Part model, mm, in its own coordinate system. Face numbers are marked on the shaded views. A direction names the side the tool comes from. Round coordinates to 2 decimals unless told otherwise and drop trailing zeros. Write each loop counter-clockwise with the first axis right and the second up, starting at its lowest first coordinate (ties: lowest second). Pieces come first, ordered by that corner, then holes.
1) Saw through at D-D on y = 13. Write the cut outline in (x, z), and give its area (3 significant figures).
2) Drill centre lines: L1, parallel to X at y = 6.75, z = 16; L2, parallel to Y at x = 5.15, z = 23; L3, parallel to Y at x = -7.9, z = 23. Where is each one in solid material? Low to high.
3) Saw through at A-A on y = 8.5. Write the cut outline in (x, z).
4) Saw through at B-B on x = 0. Write the cut outline in (y, z).
5) Which spindle directions (+Z, -Z, +X, -X, +Y, -Y) get a long thin tool onto all of the face, cutting with end or side? Do the marked faces 4, 5, 6, 7 and 8. Say none if no direction does.
6) Saw through at C-C on z = 8.5. Write the cut outline in (x, y), and give its area (3 significant figures).
7) Flat gauge pins, fed straight in: pin 1 (7 mm diameter, centred on x = 0, z = 8.5, fed in from -Y); pin 2 (1.5 mm diameter, centred on x = 8, y = 13.5, fed in from -Z); pin 3 (2 mm diameter, centred on y = 13, z = 23, fed in from -X); pin 4 (8 mm diameter, centred on x = 6.5, z = 13, fed in from +Y). Where does each tip first touch, or does it go through?
8) Pull direction X, two halves, no side cores. Call the marked faces 1, 2 and 3: +X half, -X half, draft (parallel to the pull), parting line (faces both ways), or undercut.
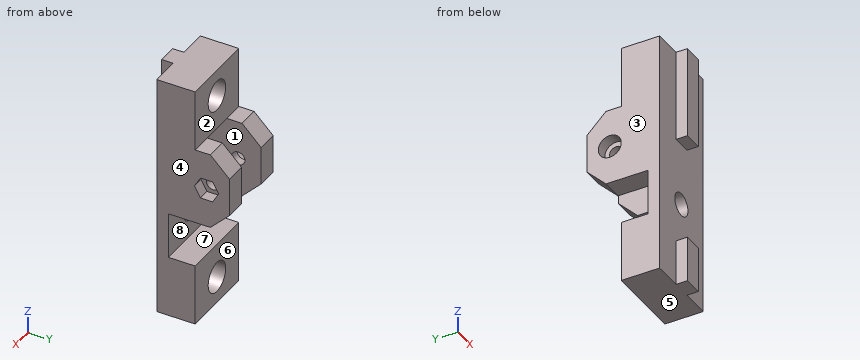
```python
from build123d import *

# Parameters (mm, degrees)
SKETCH1_W               = 20
SKETCH1_H               = 30
BOSS_EXTRUDE1_DEPTH     = 3
SKETCH2_W               = 5
SKETCH2_H               = 12
BOSS_EXTRUDE2_DEPTH     = 3
SKETCH3_R               = 7
SKETCH3_R_2             = 4
BOSS_EXTRUDE3_DEPTH     = 7
SKETCH4_R               = 4
BOSS_EXTRUDE4_DEPTH     = 1
CUT_EXTRUDE1_DEPTH      = 20.339079606
CUT_EXTRUDE1_DEPTH_BACK = 20.339079606
SKETCH5_R               = 3
SKETCH6_R               = 7
SKETCH6_R_2             = 4
BOSS_EXTRUDE6_DEPTH     = 7
SKETCH7_W               = 20
SKETCH7_H               = 3
BOSS_EXTRUDE7_DEPTH     = 19
SKETCH8_W               = 5
SKETCH8_H               = 3
BOSS_EXTRUDE8_DEPTH     = 12
SKETCH10_W              = 5.5
SKETCH10_H              = 20
BOSS_EXTRUDE9_DEPTH     = 16
CUT_EXTRUDE2_DEPTH      = 57.231663678
CUT_EXTRUDE2_DEPTH_BACK = 57.231663678
SKETCH11_R              = 1.75
SKETCH12_R              = 3
SKETCH12_R_2            = 1.75
CUT_EXTRUDE3_DEPTH      = 3
CUT_EXTRUDE4_START      = -3
SKETCH13_R              = 1.75
CUT_EXTRUDE4_DEPTH      = 3
CHAMFER2_SIZE           = 5
CUT_EXTRUDE5_START      = -1.5
SKETCH14_R              = 4
CUT_EXTRUDE5_DEPTH      = 1.5


with BuildPart() as part:
    # Sketch1 → Boss-Extrude1 (new body)
    with BuildSketch(Plane(origin=(0, 0, 0), x_dir=(1, 0, 0), z_dir=(0, 1, 0))):
        Rectangle(SKETCH1_W, SKETCH1_H)
    boss_extrude1 = extrude(amount=BOSS_EXTRUDE1_DEPTH)

    # Sketch2 → Boss-Extrude2 (add)
    with BuildSketch(Plane.XZ):
        with Locations((0, -9)):
            Rectangle(SKETCH2_W, SKETCH2_H)
    boss_extrude2 = extrude(amount=BOSS_EXTRUDE2_DEPTH)

    # Sketch3 → Boss-Extrude3 (add)
    with BuildSketch(Plane(origin=(0, 3, 0), x_dir=(1, 0, 0), z_dir=(0, 1, 0))):
        with Locations(Location((0, 8, 0), (0, 0, 90))):
            Circle(SKETCH3_R)
        with Locations(Location((0, 8, 0), (0, 0, 270))):
            Circle(SKETCH3_R_2, mode=Mode.SUBTRACT)
    boss_extrude3 = extrude(amount=BOSS_EXTRUDE3_DEPTH)

    # Sketch4 → Boss-Extrude4 (add)
    with BuildSketch(Plane(origin=(0, 3, 0), x_dir=(1, 0, 0), z_dir=(0, 1, 0))):
        with Locations(Location((0, 8, 0), (0, 0, 270))):
            Circle(SKETCH4_R)
    boss_extrude4 = extrude(amount=BOSS_EXTRUDE4_DEPTH)

    # Sketch5 → Cut-Extrude1 (cut, two sides: drawn at the far end of the back side and taken through both)
    with BuildSketch(Plane(origin=(0, 3, 0), x_dir=(1, 0, 0), z_dir=(0, 1, 0)).offset(-CUT_EXTRUDE1_DEPTH_BACK)):
        with Locations(Location((0, -8.5, 0), (0, 0, 90))):
            Circle(SKETCH5_R)
    extrude(amount=CUT_EXTRUDE1_DEPTH + CUT_EXTRUDE1_DEPTH_BACK, mode=Mode.SUBTRACT)

    # Sketch6 → Boss-Extrude6 (add)
    # profile 1 of 2: a face of its own
    with BuildSketch(Plane(origin=(0, 3, 0), x_dir=(1, 0, 0), z_dir=(0, 1, 0))):
        Polygon((0, 15), (-10, 15), (-10, -1), (10, -1), (10, 15), align=None)
        with BuildLine():
            ThreePointArc((7, 8), (-4.949747468, 3.050252532), (0, 15))
            ThreePointArc((0, 15), (4.949747468, 12.949747468), (7, 8))
        make_face(mode=Mode.SUBTRACT)
    # profile 2 of 2: a face of its own
    with BuildSketch(Plane(origin=(0, 3, 0), x_dir=(1, 0, 0), z_dir=(0, 1, 0))):
        with Locations((0, 8)):
            Circle(SKETCH6_R)
        with Locations(Location((0, 8, 0), (0, 0, 270))):
            Circle(SKETCH6_R_2, mode=Mode.SUBTRACT)
    boss_extrude6 = extrude(amount=BOSS_EXTRUDE6_DEPTH)

    # Sketch7 → Boss-Extrude7 (add)
    with BuildSketch(Plane.XY.offset(15)):
        with Locations((0, 1.5)):
            Rectangle(SKETCH7_W, SKETCH7_H)
    extrude(amount=BOSS_EXTRUDE7_DEPTH)

    # Mirror3: Boss-Extrude1, Boss-Extrude2, Boss-Extrude3, Boss-Extrude4, Boss-Extrude6 across plane
    add(boss_extrude1.mirror(Plane.XY.offset(17)))
    add(boss_extrude2.mirror(Plane.XY.offset(17)))
    add(boss_extrude3.mirror(Plane.XY.offset(17)))
    add(boss_extrude4.mirror(Plane.XY.offset(17)))
    add(boss_extrude6.mirror(Plane.XY.offset(17)))

    # Sketch8 → Boss-Extrude8 (add)
    with BuildSketch(Plane(origin=(0, 0, 37), x_dir=(-1, 0, 0), z_dir=(0, 0, -1))):
        with Locations((0, -1.5)):
            Rectangle(SKETCH8_W, SKETCH8_H)
    extrude(amount=BOSS_EXTRUDE8_DEPTH)

    # Sketch10 → Boss-Extrude9 (add)
    with BuildSketch(Plane(origin=(0, 3, 0), x_dir=(1, 0, 0), z_dir=(0, 1, 0))):
        with Locations((-7.25, -23)):
            Rectangle(SKETCH10_W, SKETCH10_H)
        with Locations((7.25, -23)):
            Rectangle(SKETCH10_W, SKETCH10_H)
    extrude(amount=BOSS_EXTRUDE9_DEPTH)

    # Sketch11 → Cut-Extrude2 (cut, two sides: drawn at the far end of the back side and taken through both)
    with BuildSketch(Plane.ZY.offset(10).offset(-CUT_EXTRUDE2_DEPTH_BACK)):
        with Locations((23, 13)):
            Circle(SKETCH11_R)
    extrude(amount=CUT_EXTRUDE2_DEPTH + CUT_EXTRUDE2_DEPTH_BACK, mode=Mode.SUBTRACT)

    # Sketch12 → Cut-Extrude3 (cut)
    with BuildSketch(Plane.ZY.offset(10)):
        with Locations((23, 13)):
            Circle(SKETCH12_R)
        with Locations((23, 13)):
            Circle(SKETCH12_R_2, mode=Mode.SUBTRACT)
    extrude(amount=-CUT_EXTRUDE3_DEPTH, mode=Mode.SUBTRACT)

    # Sketch13 → Cut-Extrude4 (cut)
    with BuildSketch(Plane(origin=(10, 0, 0), x_dir=(0, 0, -1), z_dir=(1, 0, 0)).offset(CUT_EXTRUDE4_START)):
        Polygon((-23, 16.175426481), (-25.75, 14.58771324), (-25.75, 11.41228676), (-23, 9.824573519), (-20.25, 11.41228676), (-20.25, 14.58771324), align=None)
        with Locations((-23, 13)):
            Circle(SKETCH13_R, mode=Mode.SUBTRACT)
    extrude(amount=CUT_EXTRUDE4_DEPTH, mode=Mode.SUBTRACT)

    # Chamfer2
    chamfer2_edges = [part.edges().sort_by_distance(p)[0] for p in [
        (-7.25, 19, 13),
        (-7.25, 19, 33),
        (7.25, 19, 13),
        (7.25, 19, 33),
    ]]
    chamfer(chamfer2_edges, length=CHAMFER2_SIZE)

    # Sketch14 → Cut-Extrude5 (cut)
    with BuildSketch(Plane(origin=(0, 4, 0), x_dir=(1, 0, 0), z_dir=(0, 1, 0)).offset(CUT_EXTRUDE5_START)):
        with Locations(Location((0, -42, 0), (0, 0, 90))):
            Circle(SKETCH14_R)
        with Locations(Location((0, 8, 0), (0, 0, 270))):
            Circle(SKETCH14_R)
    extrude(amount=CUT_EXTRUDE5_DEPTH, mode=Mode.SUBTRACT)


solid = part.part
```
Completed:
1. outline: (-10, 13) - (-4.5, 13) - (-4.5, 21.25) - (-7, 21.25) - (-7, 20) - (-10, 20) - close; (-10, 26) - (-7, 26) - (-7, 24.75) - (-4.5, 24.75) - (-4.5, 33) - (-10, 33) - close; (4.5, 13) - (10, 13) - (10, 20.25) - (7, 20.25) - (7, 21.25) - (4.5, 21.25) - close; (4.5, 24.75) - (7, 24.75) - (7, 25.75) - (10, 25.75) - (10, 33) - (4.5, 33) - close
1. area: 168 mm2
2. L1: x = -10 to -4.5, 4.5 to 10
2. L2: y = 0 to 11.25, 14.75 to 19
2. L3: y = 0 to 10, 16 to 19
3. outline: (-10, -15) - (10, -15) - (10, 1) - (-10, 1) - close; (-10, 13) - (-4.5, 13) - (-4.5, 33) - (4.5, 33) - (4.5, 13) - (10, 13) - (10, 49) - (-10, 49) - close; hole circle Ø8 at (0, -8); hole circle Ø8 at (0, 42)
4. outline: (-3, -15) - (10, -15) - (10, -12) - (2.5, -12) - (2.5, -4) - (10, -4) - (10, 1) - (3, 1) - (3, 5.5) - (0, 5.5) - (0, -3) - (-3, -3) - close; (-3, 25) - (0, 25) - (0, 11.5) - (3, 11.5) - (3, 33) - (10, 33) - (10, 38) - (2.5, 38) - (2.5, 46) - (10, 46) - (10, 49) - (-3, 49) - close
5. face 4: +Z, -Z, +X, +Y, -Y
5. face 5: -Z, +X, -X, +Y, -Y
5. face 6: -Z, +X, -X, +Y
5. face 7: +X, -X, +Y
5. face 8: +Y
6. outline: (-10, 0) - (-3, 0) - (-3, 3) - (-10, 3) - close; (3, 0) - (10, 0) - (10, 3) - (3, 3) - close
6. area: 42.0 mm2
7. pin 1: stops at y = 0
7. pin 2: stops at z = 13
7. pin 3: passes through
7. pin 4: stops at y = 18
8. face 1: undercut
8. face 2: draft
8. face 3: -X half
